from build123d import *

# Parameters (mm, degrees)
BLANKSKE_W           = 68
BLANKSKE_H           = 9
BLANK_DEPTH          = 10
TOOTHCUTSIM_DEPTH    = 70.318107302
TEETHCUTS_COUNT      = 23
TEETHCUTS_PITCH      = 3.14159265
SKETCH1_W            = 10
SKETCH1_H            = 8.592466409
BOSS_EXTRUDE1_DEPTH  = 8
SKETCH3_W            = 8
SKETCH3_H            = 10
BOSS_EXTRUDE2_DEPTH  = 4.5
SKETCH4_W            = 8
SKETCH4_H            = 3.8
BOSS_EXTRUDE3_DEPTH  = 8
SKETCH5_W            = 10
SKETCH5_H            = 11.170580006
CUT_EXTRUDE1_DEPTH   = 8
CUT_EXTRUDE2_DEPTH   = 1
BOSS_EXTRUDE5_DEPTH  = 0.5
FILLET8_START        = -10
FILLET8_DEPTH        = 9
FILLET8_START_2      = -18
FILLET8_2_DEPTH      = 8.45342
BOSS_EXTRUDE6_DEPTH  = 17.79
BOSS_EXTRUDE10_DEPTH = 1.5
FILLET15_R           = 1
SKETCH11_W           = 15.24537785
SKETCH11_H           = 13.543744844
CUT_EXTRUDE3_DEPTH   = 7
SKETCH16_W           = 61
SKETCH16_H           = 9
BOSS_EXTRUDE12_DEPTH = 1.4
FILLET19_R           = 1


with BuildPart() as part:
    # BlankSke → Blank (new body)
    with BuildSketch(Plane.XY):
        with Locations((34, 4.5)):
            Rectangle(BLANKSKE_W, BLANKSKE_H)
    extrude(amount=-BLANK_DEPTH)

    # TooCutSkeSim → ToothCutSim (cut, through all)
    with BuildSketch(Plane.XY):
        Polygon((0.44443537, 6.75), (-0.44443537, 6.75), (-1.272613241, 9.0254), (1.272613241, 9.0254), align=None)
    toothcutsim = extrude(amount=-TOOTHCUTSIM_DEPTH, mode=Mode.SUBTRACT)

    # TeethCuts: ToothCutSim ×23
    with Locations(*[(i * TEETHCUTS_PITCH, 0, 0) for i in range(1, TEETHCUTS_COUNT)]):
        add(toothcutsim, mode=Mode.SUBTRACT)

    # Sketch1 → Boss-Extrude1 (add)
    with BuildSketch(Plane(origin=(68, 0, 0), x_dir=(0, 0, -1), z_dir=(1, 0, 0))):
        with Locations((5, 4.296233205)):
            Rectangle(SKETCH1_W, SKETCH1_H)
    extrude(amount=BOSS_EXTRUDE1_DEPTH)

    # Sketch3 → Boss-Extrude2 (add)
    with BuildSketch(Plane(origin=(0, 8.592466409, 0), x_dir=(1, 0, 0), z_dir=(0, 1, 0))):
        with Locations((72, 5)):
            Rectangle(SKETCH3_W, SKETCH3_H)
    extrude(amount=BOSS_EXTRUDE2_DEPTH)

    # Sketch4 → Boss-Extrude3 (add)
    with BuildSketch(Plane(origin=(0, 0, -10), x_dir=(-1, 0, 0), z_dir=(0, 0, -1))):
        with Locations((-72, 11.192466409)):
            Rectangle(SKETCH4_W, SKETCH4_H)
    extrude(amount=BOSS_EXTRUDE3_DEPTH)

    # Sketch5 → Cut-Extrude1 (cut)
    with BuildSketch(Plane.ZY):
        with Locations((-5, 5.585290003)):
            Rectangle(SKETCH5_W, SKETCH5_H)
    extrude(amount=-CUT_EXTRUDE1_DEPTH, mode=Mode.SUBTRACT)

    # Sketch6 → Cut-Extrude2 (cut)
    with BuildSketch(Plane.XY):
        Polygon((8.161409553, 9), (8, 9), (8, 0), (76, 0), (76, 13.092466409), (68, 13.092466409), (68, 8.592466409), (67.851669903, 9), (67.236814047, 9), (66.41788102, 6.75), (65.52901028, 6.75), (64.710077253, 9), (64.095221397, 9), (63.27628837, 6.75), (62.38741763, 6.75), (61.568484603, 9), (60.953628747, 9), (60.13469572, 6.75), (59.24582498, 6.75), (58.426891953, 9), (57.812036097, 9), (56.99310307, 6.75), (56.10423233, 6.75), (55.285299303, 9), (54.670443447, 9), (53.85151042, 6.75), (52.96263968, 6.75), (52.143706653, 9), (51.528850797, 9), (50.70991777, 6.75), (49.82104703, 6.75), (49.002114003, 9), (48.387258147, 9), (47.56832512, 6.75), (46.67945438, 6.75), (45.860521353, 9), (45.245665497, 9), (44.42673247, 6.75), (43.53786173, 6.75), (42.718928703, 9), (42.104072847, 9), (41.28513982, 6.75), (40.39626908, 6.75), (39.577336053, 9), (38.962480197, 9), (38.14354717, 6.75), (37.25467643, 6.75), (36.435743403, 9), (35.820887547, 9), (35.00195452, 6.75), (34.11308378, 6.75), (33.294150753, 9), (32.679294897, 9), (31.86036187, 6.75), (30.97149113, 6.75), (30.152558103, 9), (29.537702247, 9), (28.71876922, 6.75), (27.82989848, 6.75), (27.010965453, 9), (26.396109597, 9), (25.57717657, 6.75), (24.68830583, 6.75), (23.869372803, 9), (23.254516947, 9), (22.43558392, 6.75), (21.54671318, 6.75), (20.727780153, 9), (20.112924297, 9), (19.29399127, 6.75), (18.40512053, 6.75), (17.586187503, 9), (16.971331647, 9), (16.15239862, 6.75), (15.26352788, 6.75), (14.444594853, 9), (13.829738997, 9), (13.01080597, 6.75), (12.12193523, 6.75), (11.303002203, 9), (10.688146347, 9), (9.86921332, 6.75), (8.98034258, 6.75), align=None)
    extrude(amount=-CUT_EXTRUDE2_DEPTH, mode=Mode.SUBTRACT)

    # Sketch7 → Boss-Extrude5 (add)
    with BuildSketch(Plane.XY.offset(-1)):
        Polygon((8.8, 0.9), (75.2, 0.9), (76, 0.9), (76, 2.9), (75.2, 2.9), (8.8, 2.9), (8, 2.9), (8, 0.9), align=None)
    boss_extrude5 = extrude(amount=BOSS_EXTRUDE5_DEPTH)

    # Mirror3: Boss-Extrude5 across plane
    add(boss_extrude5.mirror(Plane.XY.offset(-5.5)))

    # Fillet8: read off the stored shape, not the designer's step
    # Fillet8 outline → Fillet8 (add)
    with BuildSketch(Plane.XY.offset(FILLET8_START)):
        with BuildLine():
            ThreePointArc((68, 9.524078597), (67.962203176, 9.251745991), (67.851669903, 9))
            Line((67.851669903, 9), (68, 8.592466409))
            Line((68, 8.592466409), (68, 9.524078597))
        make_face()
    extrude(amount=FILLET8_DEPTH)

    # Fillet8 2 outline → Fillet8 2 (add)
    with BuildSketch(Plane.XY.offset(FILLET8_START_2)):
        with BuildLine():
            Line((68, 9.292466409), (68, 9.524078597))
            ThreePointArc((68, 9.524078597), (67.993178786, 9.407477139), (67.9728082, 9.292466409))
            Line((67.9728082, 9.292466409), (68, 9.292466409))
        make_face()
    extrude(amount=FILLET8_2_DEPTH)

    # Sketch8 → Boss-Extrude6 (add)
    with BuildSketch(Plane(origin=(0, 13.092466409, 0), x_dir=(1, 0, 0), z_dir=(0, 1, 0))):
        with BuildLine():
            Line((75, 18), (75, 21.850371294))
            ThreePointArc((75, 21.850371294), (74.998770766, 21.899938995), (74.995086086, 21.949384835))
            Line((74.995086086, 21.949384835), (73.089650394, 41.099013541))
            ThreePointArc((73.089650394, 41.099013541), (72.765752232, 41.741287239), (72.094564308, 42))
            Line((72.094564308, 42), (62.094564308, 42))
            Line((62.094564308, 42), (62.094564308, 30))
            Line((62.094564308, 30), (64.933441114, 30))
            Line((64.933441114, 30), (68.447653948, 30))
            ThreePointArc((68.447653948, 30), (69.169019838, 29.692554151), (69.446823832, 28.959262504))
            Line((69.446823832, 28.959262504), (69, 18))
            Line((69, 18), (75, 18))
        make_face()
    extrude(amount=-BOSS_EXTRUDE6_DEPTH)

    # Sketch14 → Boss-Extrude10 (add)
    with BuildSketch(Plane.XZ.offset(-9.292466409)):
        Polygon((76, -10), (67.9728082, -10), (67.9728082, -18), (69, -18), (75, -18), (76, -18), align=None)
    extrude(amount=BOSS_EXTRUDE10_DEPTH)

    # Fillet15
    fillet15_edges = [part.edges().sort_by_distance(p)[0] for p in [
        (71.9864041, 7.792466409, -10),
        (72, 7.792466409, -18),
    ]]
    fillet(fillet15_edges, radius=FILLET15_R)

    # Sketch11 → Cut-Extrude3 (cut)
    with BuildSketch(Plane.ZY.offset(-8)):
        with Locations((-5.226368624, 3.937583059)):
            Rectangle(SKETCH11_W, SKETCH11_H)
    extrude(amount=-CUT_EXTRUDE3_DEPTH, mode=Mode.SUBTRACT)

    # Sketch16 → Boss-Extrude12 (add)
    with BuildSketch(Plane.XZ):
        with Locations((45.5, -5.5)):
            Rectangle(SKETCH16_W, SKETCH16_H)
    extrude(amount=BOSS_EXTRUDE12_DEPTH)

    # Fillet19
    fillet19_edges = [part.edges().sort_by_distance(p)[0] for p in [
        (75, 10.442466409, -18),
        (69, 10.442466409, -18),
    ]]
    fillet(fillet19_edges, radius=FILLET19_R - 0.0001)  # a hair under: the kernel refuses the full size


solid = part.part
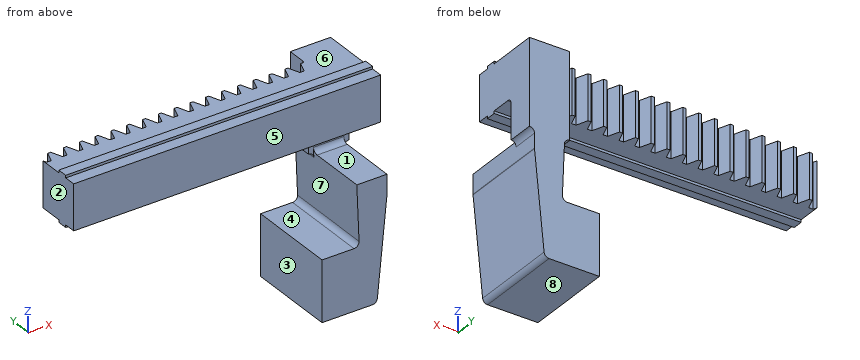
For this review, take the finished solid that the model builds, in its own axes (mm). Face numbers are marked on the shaded views. A direction names the side the tool comes from. Round coordinates to 2 decimals unless told otherwise and drop trailing zeros. Order: outer loops, then holes, each group sorted by start corner. A loop starts at its lowest first (then second) coordinate and runs counter-clockwise, first axis right, second up. Notation, with made-up numbers: (10.25, -35.5) -> (31.25, -35.5) arc R7 ccw to (31.25, -25.5) -> close; hole circle Ø11 at (74.25, 10.5). An arc over 180 degrees is marked (long way). Put each result on its own line as item: value.
Q1. Add section D-D on z = -26.5. Write out the cut boundary in (x, y), plus the area to 3 significant figures.
Check result:
outline: (69.35, -4.7) -> (74.54, -4.7) -> (74.54, 13.09) -> (69.35, 13.09) -> close
area: 92.4 mm2
Q2. Add section B-B on y = -2.5. Write out the cut boundary in (x, z), plus the area to 3 significant figures.
Check result:
outline: (62.09, -42) -> (72.09, -42) arc R1 ccw to (73.09, -41.1) -> (75, -21.95) arc R1 ccw to (75, -21.85) -> (75, -18) -> (69, -18) -> (69.45, -28.96) arc R1 cw to (68.45, -30) -> (62.09, -30) -> close
area: 204 mm2
Q3. Machinability: for the marked faces 1, 2, 3, 4 and 5, which of the approach directions +Z, -Z, +X, -X, +Y, -Y give a long, thin tool a straight path to every point of the face, cutting with its end or side? Answer none if there is none.
Check result:
face 1: +X, -X, -Y
face 2: +Z, -Z, -X, +Y, -Y
face 3: -Z, -X, +Y, -Y
face 4: -X, +Y, -Y
face 5: +Z, +X, -X, -Y
Q4. Mouldability with a two-part tool opening along Z and no side actions: class the marked faces 6, 7 and 8 as pulls with the +Z half, pulls with the -Z half, needs draft (parallel to the pull), parting line crosses it, or undercut.
Check result:
face 6: pulls with the +Z half
face 7: undercut
face 8: pulls with the -Z half
Q5. For probe 1 along Z at (x, y) = (69.5, 8.25); probe 2 along Z at (x, y) = (21, 0); probe 3 along X at (y, z) = (10.5, -12), list the stretches that pass through material, from the lowest coordinate up. Write a range as [from, to].
Check result:
probe 1: [-42, -1]
probe 2: [-10, -1]
probe 3: [68, 76]
Q6. Add section A-A on y = 5.5. Write out the cut boundary in (x, z).
Check result:
outline: (15, -10) -> (76, -10) -> (76, -1) -> (15, -1) -> close; (62.09, -42) -> (72.09, -42) arc R1 ccw to (73.09, -41.1) -> (75, -21.95) arc R1 ccw to (75, -21.85) -> (75, -18) -> (69, -18) -> (69.45, -28.96) arc R1 cw to (68.45, -30) -> (62.09, -30) -> close
Q7. Add section C-C on z = -15. Write out the cut boundary in (x, y), plus the area to 3 significant figures.
Check result:
outline: (67.97, 7.79) -> (76, 7.79) -> (76, 13.09) -> (68, 13.09) -> (68, 9.52) arc R1 cw to (67.97, 9.29) -> close
area: 42.4 mm2
Q8. Insertion check: pin 1 Ø6 at (x, z) = (62, -11) entering from +Y; pin 2 Ø1 at (x, y) = (62, -0.5) entering from +Z; pin 3 Ø5.5 at (y, z) = (1, -18.5) entering from +X. Each pin has a flat end and moves straight along its axis. Give the tip position at first contact, or say it passes through.
Check result:
pin 1: y = 9
pin 2: z = -1
pin 3: x = 75
